Autodesk Inventor part; units mm, degrees
ref_plane "YZ Plane" through (0, 0, 0) normal (1, 0, 0) x (0, 1, 0)
ref_plane "XZ Plane" through (0, 0, 0) normal (0, 1, 0) x (-1, 0, 0)
ref_plane "XY Plane" through (0, 0, 0) normal (0, 0, 1) x (1, 0, 0)
sketch "Sketch1" plane through (0, 0, 0) normal (0, 1, 0) x (-1, 0, 0)
  line L0 (0, 0) -> (-43, 0)
  line L1 (-43, 0) -> (-43, -48)
  line L2 (-43, -48) -> (0, -48)
  line L3 (0, -48) -> (0, 0)
  circle A0 centre (-21.5, -22) radius 2
  point P0 (-43, -24)
  point P1 (-21.5, -48)
  dimension "d0" = 43
  dimension "d1" = 48
  dimension "d2" = 4
  dimension "d23" = 22
extrude "Extrusion1" add sketch "Sketch1" along normal blind 13
sketch "Sketch2" plane through (0, 13, 0) normal (0, 1, 0) x (1, 0, 0)
  line L0 (11.5, 54.8346) -> (31.5, 54.8346)
  line L1 (31.5, 54.8346) -> (31.5, -5.4848)
  line L2 (31.5, -5.4848) -> (11.5, -5.4848)
  line L3 (11.5, -5.4848) -> (11.5, 54.8346)
  line L4 (43, 48) -> (0, 48)
  point P0 (0, 0)
  point P1 (21.5, 54.8346)
  point P2 (21.5, 48)
  dimension "d5" = 20
extrude "Extrusion2" cut sketch "Sketch2" against normal blind 3
sketch "Sketch3" plane through (0, 0, 0) normal (0, -1, 0) x (1, 0, 0)
  line L0 (23.5207, -18.5) -> (25.5415, -22)
  line L1 (25.5415, -22) -> (23.5207, -25.5)
  line L2 (23.5207, -25.5) -> (19.4793, -25.5)
  line L3 (19.4793, -25.5) -> (17.4585, -22)
  line L4 (17.4585, -22) -> (19.4793, -18.5)
  line L5 (19.4793, -18.5) -> (23.5207, -18.5)
  line L6 (43, -48) -> (0, -48)
  line L7 (0, -48) -> (0, 0)
  line L8 (0, 0) -> (43, 0)
  point P0 (21.5, -22)
  point P1 (21.5, -25.5)
  point P2 (21.5, -48)
  point P3 (0, -24)
  dimension "d8" = 7
  dimension "d24" = 22
extrude "Extrusion3" cut sketch "Sketch3" against normal blind 5
sketch "Sketch4" plane through (43, 0, 0) normal (1, 0, 0) x (0, 0, -1)
  circle A0 centre (24, 5.5) radius 2
  circle A1 centre (32, 5.5) radius 2
  circle A2 centre (16, 5.5) radius 2
  circle A3 centre (40, 5.5) radius 2
  circle A4 centre (8, 5.5) radius 2
  line L0 (0, 0) -> (48, 0)
  line L1 (0, 13) -> (48, 13)
  point P0 (24, 13)
  dimension "d11" = 4
  dimension "d12" = 4
  dimension "d13" = 4
  dimension "d14" = 4
  dimension "d15" = 4
  dimension "d16" = 8
  dimension "d17" = 8
  dimension "d18" = 8
  dimension "d19" = 8
  dimension "d20" = 5.5
extrude "Extrusion4" cut sketch "Sketch4" against normal through all contours A1 | A2 | A3 | A4
fillet "Fillet1" radius 1 7 edges at (11.5, 13, -24) (31.5, 13, -24) (11.5, 11.5, -48) (31.5, 11.5, -48) (37.25, 13, -48) (5.75, 13, -48) (21.5, 10, -48)
fillet "Fillet2" radius 1 15 edges at (43, 12.7071, -47.7071) (43, 6, -48) (43, 13, -23.5) (0, 12.7071, -47.7071) (0, 6, -48) (0, 13, -23.5) (11.2071, 12.7071, 0) (11.5, 11, 0) (5.25, 13, 0) (31.7929, 12.7071, 0) (31.5, 11, 0) (37.75, 13, 0) (0, 6.5, 0) (43, 6.5, 0) (21.5, 10, 0)
sketch "Sketch5" plane through (0, 13, 0) normal (0, 1, 0) x (1, 0, 0)
  circle A0 centre (5.5, 40) radius 2
  circle A1 centre (5.5, 8) radius 2
  line L0 (0, 47) -> (0, 1)
  line L1 (10.5, 48) -> (1, 48)
  circle A2 centre (37.5, 40) radius 2
  circle A3 centre (37.5, 8) radius 2
  line L2 (43, 1) -> (43, 47)
  point P0 (0, 0)
  dimension "d27" = 4
  dimension "d28" = 4
  dimension "d29" = 5.5
  dimension "d30" = 8
  dimension "d31" = 32
  dimension "d32" = 4
  dimension "d33" = 4
  dimension "d34" = 5.5
extrude "Extrusion5" cut sketch "Sketch5" against normal through all
sketch "Sketch6" plane through (0, 13, 0) normal (0, 1, 0) x (1, 0, 0)
  circle A0 centre (5.5, 40) radius 3.6
  circle A1 centre (5.5, 8) radius 3.6
  circle A2 centre (37.5, 40) radius 3.6
  circle A3 centre (37.5, 8) radius 3.6
  circle A4 centre (37.5, 40) radius 2
  circle A5 centre (37.5, 8) radius 2
  circle A6 centre (5.5, 8) radius 2
  circle A7 centre (5.5, 40) radius 2
  point P0 (0, 0)
  dimension "d37" = 7.2
  dimension "d38" = 7.2
  dimension "d39" = 7.2
  dimension "d40" = 7.2
extrude "Extrusion6" cut sketch "Sketch6" against normal blind 3
properties part number "slidescentermount"
Could you check a few things on this model? Use its own coordinates, in mm. A direction names the side the tool comes from. Coordinates: 2 decimals unless noted, no trailing zeros. Order: outer loops, then holes, each group sorted by start corner. A loop starts at its lowest first (then second) coordinate and runs counter-clockwise, first axis right, second up. Notation, with made-up numbers: M 29.25,38 L 56.25,38 A7 ccw 56.25,46 Z; hole C 80.5,32 d6. An arc over 180 degrees is marked long. Use one line per item in the form item = value. Start each with the question number.
1. We'd pull the mould along X, two halves only. Please class faces 1 (the cylindrical face through (31.785, 10.812, -47.699)), 2 (the cylindrical face through (21.724, 5.588, -6.002)), 3 (the cylindrical face through (42.715, 12.699, -23.678)): +X half, -X half, draft (parallel to the pull), parting line (faces both ways), or undercut.
2. Suppose I cut it at C-C on x = 30. Write out the boundary of the cut face in (y, z).
3. Suppose I cut it at A-A on z = -16. Write out the boundary of the cut face in (x, y), then the cut area to 3 significant figures.
4. On a 3-axis mill with a long thin cutter (end or side, diameter ignored), from which of +Z, -Z, +X, -X, +Y, -Y can I reach the whole of each face in a straight line? I mean faces 4 (the cylindrical face through (37.03, 11.52, -43.57)), 5 (the flat face through (22, 2, -25.5)), 6 (the flat face through (11.5, 11, -24)). Say none if no direction works.
5. Suppose I cut it at B-B on x = 22. Write out the boundary of the cut face in (y, z).
6. For pin 1 (4.5 mm diameter, centred on x = 5.5, z = -40, fed in from +Y), with a flat end and sliding along its axis, tell me the tip position at first contact or that it passes through.
7. Please list where these lines run through material, in increasing order: line 1 (X direction, y = 12, z = -37); line 2 (Z direction, x = 37.5, y = 2.3); line 3 (Z direction, x = 5.5, y = 11.9).
8. Suppose I cut it at D-D on z = -27.5. Write out the boundary of the cut face in (x, y), then the cut area to 3 significant figures.
Geometry says:
q1.face_1 = undercut
q1.face_2 = draft
q1.face_3 = +X half
q2.outline = M 0,-48 L 9,-48 A1 ccw 10,-47 L 10,-1 A1 ccw 9,0 L 0,0 Z; hole C 5.5,-40 d4; hole C 5.5,-32 d4; hole C 5.5,-16 d4; hole C 5.5,-8 d4
q3.outline = M 0,0 L 43,0 L 43,3.5 L 0,3.5 Z; M 0,7.5 L 43,7.5 L 43,12 A1 ccw 42,13 L 32.5,13 A1 ccw 31.5,12 L 31.5,10 L 11.5,10 L 11.5,12 A1 ccw 10.5,13 L 1,13 A1 ccw 0,12 Z
q3.area = 326 mm^2
q4.face_4 = +Y
q4.face_5 = -Y
q4.face_6 = +Z, -Z, +Y
q5.outline = M 0,-48 L 9,-48 A1 ccw 10,-47 L 10,-23.94 L 5,-23.94 L 5,-25.5 L 0,-25.5 Z; M 0,-18.5 L 5,-18.5 L 5,-20.06 L 10,-20.06 L 10,-1 A1 ccw 9,0 L 0,0 Z; hole C 5.5,-40 d4; hole C 5.5,-32 d4; hole C 5.5,-16 d4; hole C 5.5,-8 d4
q6.pin_1 = 10
q7.line_1 = 0 to 3.51, 7.49 to 11.5, 31.5 to 35.51, 39.49 to 43
q7.line_2 = -48 to -42, -38 to -10, -6 to 0
q7.line_3 = -48 to -43.6, -36.4 to -11.6, -4.4 to 0
q8.outline = M 0,0 L 43,0 L 43,12 A1 ccw 42,13 L 32.5,13 A1 ccw 31.5,12 L 31.5,10 L 11.5,10 L 11.5,12 A1 ccw 10.5,13 L 1,13 A1 ccw 0,12 Z
q8.area = 498 mm^2
